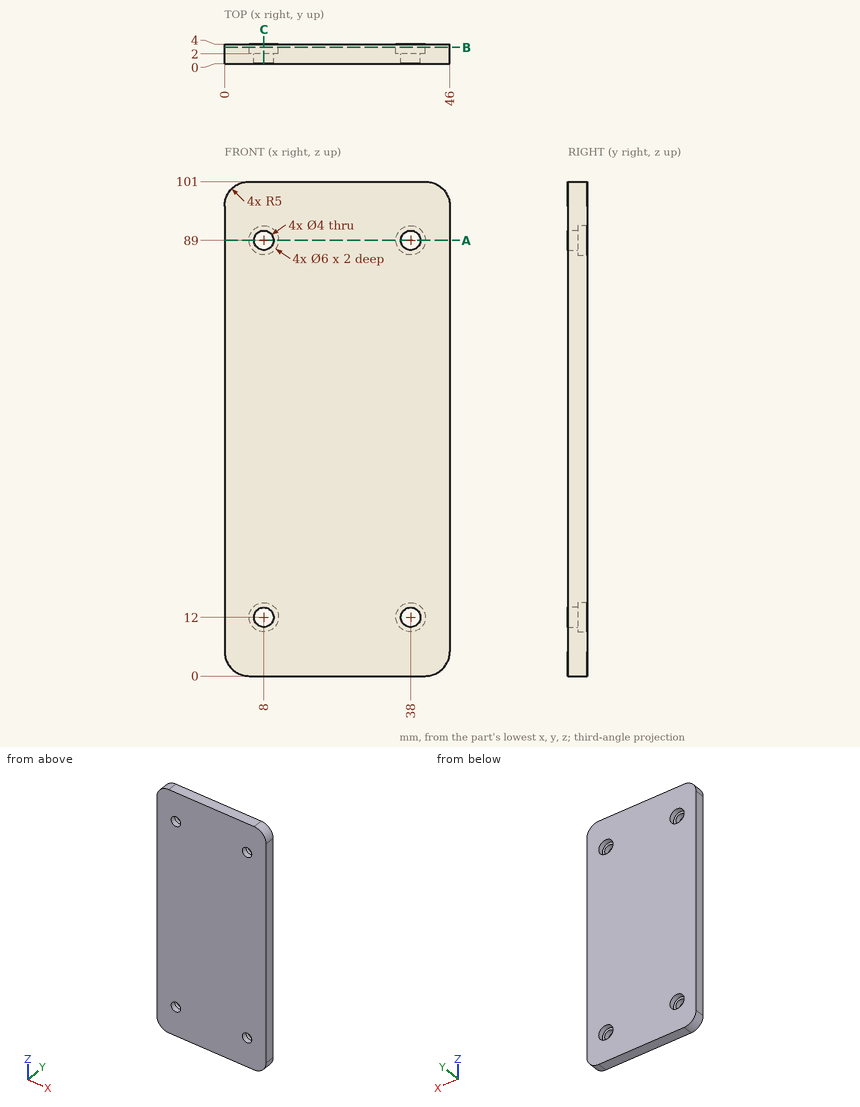
Check sheet for the drawn part. Datum: minimum x, y, z corner. Units: mm. Coordinates: 2 decimals unless noted, no trailing zeros. Loops run counter-clockwise (first coordinate to the right, second up) from the corner with the lowest first, then second, coordinate; pieces in that order, holes last. Notation, with made-up numbers: (-17, 83) -> (18, 83) arc R30 cw to (18, 114) -> close; hole circle Ø5 at (-34, 78.5). An arc over 180 degrees is marked (long way). Answer in a Markdown table with one row per item.
1. Sectioned sample at C-C, the plane x = 8. Record the boundary of the cut face in (y, z).
Check values:
| item | result |
|---|---|
| outline | (0, 0) -> (4, 0) -> (4, 9) -> (2, 9) -> (2, 10) -> (0, 10) -> close; (0, 14) -> (2, 14) -> (2, 15) -> (4, 15) -> (4, 86) -> (2, 86) -> (2, 87) -> (0, 87) -> close; (0, 91) -> (2, 91) -> (2, 92) -> (4, 92) -> (4, 101) -> (0, 101) -> close |
2. Sectioned sample at B-B, the plane y = 3.3. Record the boundary of the cut face in (x, z), then the cut area to 3 significant figures.
Check values:
| item | result |
|---|---|
| outline | (0, 5) arc R5 ccw to (5, 0) -> (41, 0) arc R5 ccw to (46, 5) -> (46, 96) arc R5 ccw to (41, 101) -> (5, 101) arc R5 ccw to (0, 96) -> close; hole circle Ø6 at (8, 12); hole circle Ø6 at (8, 89); hole circle Ø6 at (38, 12); hole circle Ø6 at (38, 89) |
| area | 4,510 mm2 |
3. Go/stop test with flat-tipped pins: pin 1 (8 mm diameter, centred on x = 8, z = 12, fed in from -Y); pin 2 (5 mm diameter, centred on x = 8, z = 89, fed in from +Y). Record where each tip stops, or that it passes through.
Check values:
| item | result |
|---|---|
| pin 1 | stops at y = 0 |
| pin 2 | stops at y = 2 |
4. Material ranges on line 1 along X through (y, z) = (0.75, 89); line 2 along X through (y, z) = (2.6, 14); line 3 along Z through (x, y) = (6.5, 1.05), recorded low to high. Write a range as [from, to].
Check values:
| item | result |
|---|---|
| line 1 | x = [0, 6], [10, 36], [40, 46] |
| line 2 | x = [0, 5.76], [10.24, 35.76], [40.24, 46] |
| line 3 | z = [0, 10.68], [13.32, 87.68], [90.32, 101] |
5. Sectioned sample at A-A, the plane z = 89. Record the boundary of the cut face in (x, y), then the cut area to 3 significant figures.
Check values:
| item | result |
|---|---|
| outline | (0, 0) -> (6, 0) -> (6, 2) -> (5, 2) -> (5, 4) -> (0, 4) -> close; (10, 0) -> (36, 0) -> (36, 2) -> (35, 2) -> (35, 4) -> (11, 4) -> (11, 2) -> (10, 2) -> close; (40, 0) -> (46, 0) -> (46, 4) -> (41, 4) -> (41, 2) -> (40, 2) -> close |
| area | 144 mm2 |
